For this review, take the finished solid that the model builds, in its own axes (mm). Round coordinates to 2 decimals unless told otherwise and drop trailing zeros. Write each loop counter-clockwise with the first axis right and the second up, starting at its lowest first coordinate (ties: lowest second). Pieces come first, ordered by that corner, then holes. Notation, with made-up numbers: M 60.25,50.25 L 111.25,50.25 A15 ccw 111.25,78.25 Z; hole C 53,56.5 d8. An arc over 180 degrees is marked long. Use one line per item in the form item = value. Start each with the question number.
Item 1: Add section A-A (z = 0). State the section outline as (x, y) points, and give its area (3 significant figures).
Item 2: Add section B-B (x = 9). State the section outline as (y, z) points.
Item 3: Draft analysis for pull direction Z (two halves, no side actions). For faces 1 (the cylindrical face through (25.861, 2.465, 5.745)), 2 (the flat face through (14, 2, -8)), 3 (the conical face through (11.55, 2.58, 0.8)), 4 (the cylindrical face through (6.5, 3.9, 0.1)), state which applies: released by +Z, released by -Z, zero draft, split by the parting line, or undercut.
Item 4: Add section C-C (y = 4.25). State the section outline as (x, z) points.
Item 5: Add section D-D (x = 21). State the section outline as (y, z) points.
Item 6: For line 1 (X direction, y = 0.85, z = -0.25); line 2 (X direction, y = 0.6, z = 0.25); line 3 (Z direction, x = 9, y = 3.55), list the stretches that pass through material, from the lowest coordinate up. Write a range as [from, to].
Item 7: For P1, Ø8, axis at x = 9, z = 0, coming from the -Y side; P2, Ø4.5, axis at x = 21, z = 0, coming from the +Y side; P3, Ø3, axis at y = 3.5, z = 4.5, coming from the -X side; P4, Ø1.5, axis at x = 24.5, z = 1.5, coming from the +Y side, all flat-tipped, find the tip position at first contact; note any pin that passes through.
Autodesk Inventor part; units mm, degrees
ref_plane "frame_bolt_XY" through (21, 2.25, 0) normal (0, 1, 0) x (1, 0, 0)
ref_plane "frame_bolt_YZ" through (21, 2.25, 0) normal (1, 0, 0) x (0, 0, -1)
ref_plane "frame_bolt_ZX" through (21, 2.25, 0) normal (0, 0, -1) x (0, 1, 0)
sketch "Sketch_1" plane through (0, 0, 0) normal (0, 0, 1) x (1, 0, 0)
  line L0 (0, 0) -> (28, 0)
  line L1 (28, 0) -> (28, 3.5)
  arc A0 (28, 3.5) -> (26.5, 5) centre (26.5, 3.5) ccw
  line L2 (26.5, 5) -> (1.5, 5)
  arc A1 (1.5, 5) -> (0, 3.5) centre (1.5, 3.5) ccw
  line L3 (0, 3.5) -> (0, 0)
extrude "Extrusion1" add sketch "Sketch_1" along normal mid plane 16
sketch "Sketch_2" plane through (0, 0, 0) normal (1, 0, 0) x (0, 1, 0)
  line L0 (14.3017, 20.7284) -> (-9.9569, 20.7284)
  line L1 (-9.9569, 20.7284) -> (-9.9569, -18.375)
  line L2 (-9.9569, -18.375) -> (14.3017, -18.375)
  line L3 (14.3017, -18.375) -> (14.3017, 20.7284)
  line L4 (0, 8) -> (0, -8)
  line L5 (0, -8) -> (3.5, -8)
  arc A0 (3.5, -8) -> (5, -6.5) centre (3.5, -6.5) ccw
  line L6 (5, -6.5) -> (5, 6.5)
  arc A1 (5, 6.5) -> (3.5, 8) centre (3.5, 6.5) ccw
  line L7 (3.5, 8) -> (0, 8)
extrude "Extrusion2" cut sketch "Sketch_2" along normal blind 28
sketch "Sketch_3" plane through (0, 0, 0) normal (0, 0, 1) x (1, 0, 0)
  line L0 (21, 0) -> (21, 5)
  line L1 (21, 5) -> (26.25, 5)
  line L2 (26.25, 5) -> (23.5, 2.25)
  line L3 (23.5, 2.25) -> (23.5, 0)
  line L4 (23.5, 0) -> (21, 0)
  line L5 (21, 0) -> (21, 5)
revolve "Revolution1" cut sketch "Sketch_3" angle 360 about axis through (21, 0, 0) along (0, -1, 0)
sketch "Sketch_4" plane through (0, 0, 0) normal (0, 0, 1) x (1, 0, 0)
  line L0 (9, 0) -> (9, 5)
  line L1 (9, 5) -> (11.5, 5)
  line L2 (11.5, 5) -> (11.5, 2.75)
  line L3 (11.5, 2.75) -> (14.25, 0)
  line L4 (14.25, 0) -> (9, 0)
  line L5 (9, 0) -> (9, 5)
revolve "Revolution2" cut sketch "Sketch_4" angle 360 about axis through (9, 0, 0) along (0, -1, 0)
sketch "Sketch_7" plane through (0, 0, 0) normal (0, 1, 0) x (-1, 0, 0)
  line L0 (14, -16) -> (14, 16)
  line L1 (14, 16) -> (-34, 16)
  line L2 (-34, 16) -> (-34, -16)
  line L3 (-34, -16) -> (14, -16)
  arc A0 (0, 0.5) -> (-7.5, 8) centre (-7.5, 0.5) ccw
  line L4 (-7.5, 8) -> (-20.5, 8)
  arc A1 (-20.5, 8) -> (-28, 0.5) centre (-20.5, 0.5) ccw
  line L5 (-28, 0.5) -> (-28, -0.5)
  arc A2 (-28, -0.5) -> (-20.5, -8) centre (-20.5, -0.5) ccw
  line L6 (-20.5, -8) -> (-7.5, -8)
  arc A3 (-7.5, -8) -> (0, -0.5) centre (-7.5, -0.5) ccw
  line L7 (0, -0.5) -> (0, 0.5)
extrude "Extrusion3" cut sketch "Sketch_7" along normal blind 5
ref_plane "frame_bolt_XY" through (21, 2.25, 0) normal (0, 1, 0) x (1, 0, 0)
ref_plane "frame_bolt_YZ" through (21, 2.25, 0) normal (1, 0, 0) x (0, 0, -1)
ref_plane "frame_bolt_ZX" through (21, 2.25, 0) normal (0, 0, -1) x (0, 1, 0)
ref_plane "pull_bolt_XY" through (9, 2.75, 0) normal (0, -1, 0) x (1, 0, 0)
ref_plane "pull_bolt_YZ" through (9, 2.75, 0) normal (1, 0, 0) x (0, 0, 1)
ref_plane "pull_bolt_ZX" through (9, 2.75, 0) normal (0, 0, 1) x (0, -1, 0)
properties part number "UWANGFplate"
Calculated:
q1.outline = M 0,0 L 3.75,0 L 6.5,2.75 L 6.5,5 L 1.5,5 A1.5 ccw 0,3.5 Z; M 11.5,2.75 L 14.25,0 L 18.5,0 L 18.5,2.25 L 15.75,5 L 11.5,5 Z; M 23.5,0 L 28,0 L 28,3.5 A1.5 ccw 26.5,5 L 26.25,5 L 23.5,2.25 Z
q1.area = 73.9 mm^2
q2.outline = M 0,-8 L 3.5,-8 A1.5 ccw 5,-6.5 L 5,-2.5 L 2.75,-2.5 L 0,-5.25 Z; M 0,5.25 L 2.75,2.5 L 5,2.5 L 5,6.5 A1.5 ccw 3.5,8 L 0,8 Z
q3.face_1 = released by +Z
q3.face_2 = released by -Z
q3.face_3 = undercut
q3.face_4 = undercut
q4.outline = M 0.2,-2.22 A7.5 ccw 5.78,-7.8 L 22.22,-7.8 A7.5 ccw 27.8,-2.22 L 27.8,2.22 A7.5 ccw 22.22,7.8 L 5.78,7.8 A7.5 ccw 0.2,2.22 Z; hole C 9,0 d5; hole C 21,0 d9
q5.outline = M 0,-7.98 L 3.72,-7.98 A1.5 ccw 5,-6.5 L 5,-5.25 L 2.25,-2.5 L 0,-2.5 Z; M 0,2.5 L 2.25,2.5 L 5,5.25 L 5,6.5 A1.5 ccw 3.72,7.98 L 0,7.98 Z
q6.line_1 = [0, 4.61], [13.39, 18.51], [23.49, 28]
q6.line_2 = [0, 4.36], [13.64, 18.51], [23.49, 28]
q6.line_3 = [-8, -2.5], [2.5, 8]
q7.P1 = 1.25
q7.P2 = through
q7.P3 = 0.43
q7.P4 = 4.31
